Study the drawing (mm; zero at the part's minimum x, y, z) and answer. Coordinates: 2 decimals unless noted, no trailing zeros. Loops run counter-clockwise (first coordinate to the right, second up) from the corner with the lowest first, then second, coordinate; pieces in that order, holes last.
Q1. Section B-B (z = 2.1) is taken. Count the separate pieces of the cut face and the enclosed holes in it, then the cut area to 3 significant figures.
Q2. Straight lines are drawn through the part: line 1 (Y direction, x = 5, z = 2.7); line 2 (Y direction, x = 4.25, z = 3.15); line 3 (Y direction, x = 9, z = 0.5). For each, find the intervals that lie inside material, in ascending order.
Q3. Section D-D (x = 9) is taken. Give the vertices of the cut face in (y, z), then the cut area to 3 significant figures.
Q4. Section C-C (x = 4) is taken. Give the vertices of the cut face in (y, z).
Q5. Section A-A (y = 90) is taken. Give the vertices of the cut face in (x, z).
Q6. Flat-ended cylindrical pins translate along their axes: P1, Ø6, axis at x = 5, y = 90, coming from the +Z side; P2, Ø4.5, axis at x = 5, y = 50, coming from the -Z side. Find the tip coordinate at first contact, or state that the pin passes through.
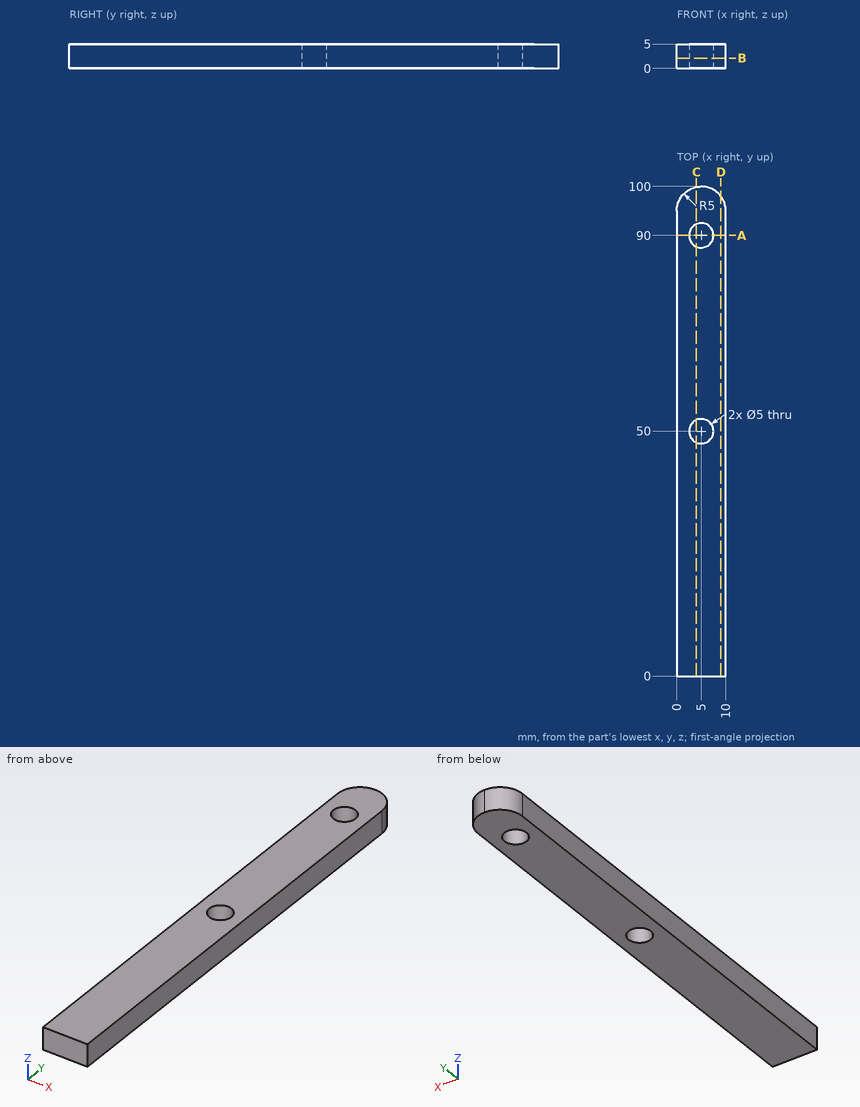
Numbers:
1. separate pieces: 1
1. enclosed holes: 2
1. area: 950 mm2
2. line 1: y = 0 to 47.5, 52.5 to 87.5, 92.5 to 100
2. line 2: y = 0 to 47.62, 52.38 to 87.62, 92.38 to 99.94
2. line 3: y = 0 to 98
3. outline: (0, 0) - (98, 0) - (98, 5) - (0, 5) - close
3. area: 490 mm2
4. outline: (0, 0) - (47.71, 0) - (47.71, 5) - (0, 5) - close; (52.29, 0) - (87.71, 0) - (87.71, 5) - (52.29, 5) - close; (92.29, 0) - (99.9, 0) - (99.9, 5) - (92.29, 5) - close
5. outline: (0, 0) - (2.5, 0) - (2.5, 5) - (0, 5) - close; (7.5, 0) - (10, 0) - (10, 5) - (7.5, 5) - close
6. P1: stops at z = 5
6. P2: passes through
